Source: three-view drawing plus pictorial views. Frame: mm from the lowest corner of the part. Give positions to 0.01 mm unless a question says otherwise; leave off trailing zeros. Order: outer loops, then holes, each group sorted by start corner. A loop starts at its lowest first (then second) coordinate and runs counter-clockwise, first axis right, second up. Notation, with made-up numbers: (17, 0) -> (39, 0) arc R23 ccw to (39, 15) -> close; hole circle Ø6 at (-36.5, -25.75). An arc over 180 degrees is marked (long way). Answer in a Markdown table with one row per item. Add a question column.
Q1. Cut plane A-A on z = 50. Return the cut outline in (x, y).
Q2. Cut plane D-D on z = 74.5. Return the cut outline in (x, y).
Q3. Contact query for flat-ended pins moving along their axis: P1, Ø8, axis at y = 5.5, z = 85, coming from the +X side; P2, Ø2, axis at x = 13, y = 11.5, coming from the +Z side; P3, Ø1.1, axis at y = 20.5, z = 50.5, coming from the -X side. Output: stop coordinate, or through.
Q4. Line query: line 1 along Y through (x, z) = (80.5, 84.5); line 2 along X through (y, z) = (16, 49.5); line 3 along Z through (x, y) = (49, 13.75). Output: solid intervals per line, ascending. Write a range as from..to.
Q5. Cut plane B-B on x = 44. Return the cut outline in (y, z).
Q6. Cut plane C-C on y = 7.5. Return the cut outline in (x, z).
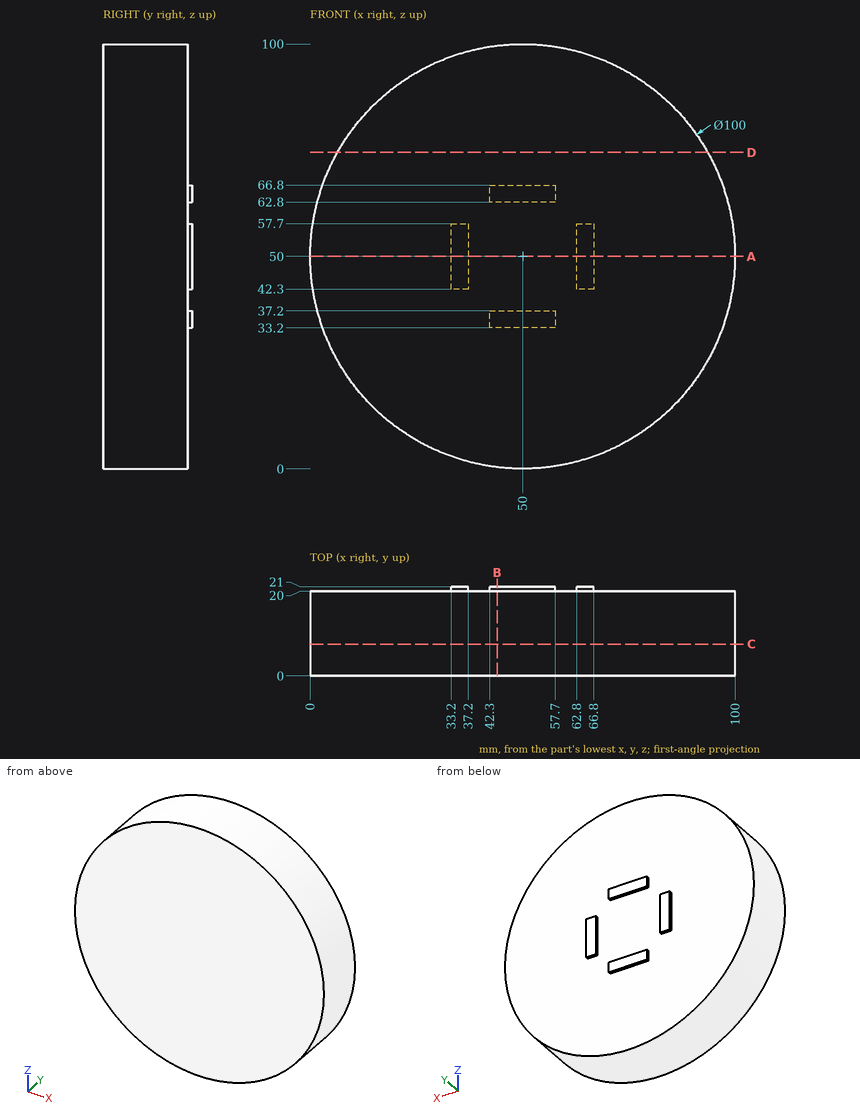
Completed:
| question | item | result |
|---|---|---|
| 1 | outline | (0, 0) -> (100, 0) -> (100, 20) -> (66.8, 20) -> (66.8, 21) -> (62.8, 21) -> (62.8, 20) -> (37.2, 20) -> (37.2, 21) -> (33.2, 21) -> (33.2, 20) -> (0, 20) -> close |
| 2 | outline | (6.41, 0) -> (93.59, 0) -> (93.59, 20) -> (6.41, 20) -> close |
| 3 | P1 | stops at x = 89.23 |
| 3 | P2 | stops at z = 84.7 |
| 3 | P3 | stops at x = 0 |
| 4 | line 1 | y = 0..20 |
| 4 | line 2 | x = 0..100 |
| 4 | line 3 | z = 0.01..99.99 |
| 5 | outline | (0, 0.36) -> (20, 0.36) -> (20, 33.2) -> (21, 33.2) -> (21, 37.2) -> (20, 37.2) -> (20, 62.8) -> (21, 62.8) -> (21, 66.8) -> (20, 66.8) -> (20, 99.64) -> (0, 99.64) -> close |
| 6 | outline | circle Ø100 at (50, 50) |
